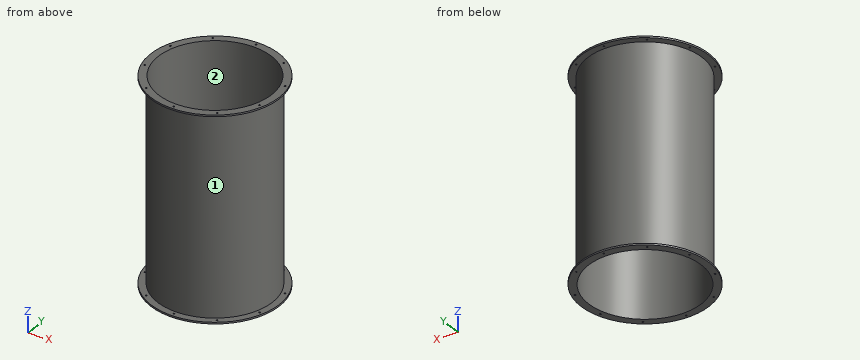
```python
from build123d import *

# Parameters (mm, degrees)
SKETCH1_R           = 425
SKETCH1_R_2         = 419
BOSS_EXTRUDE1_DEPTH = 1500
BOSS_EXTRUDE2_START = -12
SKETCH2_R           = 475
SKETCH2_R_2         = 425
BOSS_EXTRUDE2_DEPTH = 12
SKETCH4_R           = 475
SKETCH4_R_2         = 425
BOSS_EXTRUDE3_DEPTH = 12
SKETCH6_R           = 6
CUT_EXTRUDE3_DEPTH  = 1644.547991389


with BuildPart() as part:
    # Sketch1 → Boss-Extrude1 (new body)
    with BuildSketch(Plane.XY):
        Circle(SKETCH1_R)
        Circle(SKETCH1_R_2, mode=Mode.SUBTRACT)
    extrude(amount=BOSS_EXTRUDE1_DEPTH)

    # Sketch2 → Boss-Extrude2 (add)
    with BuildSketch(Plane.XY.offset(1500).offset(BOSS_EXTRUDE2_START)):
        Circle(SKETCH2_R)
        Circle(SKETCH2_R_2, mode=Mode.SUBTRACT)
    extrude(amount=BOSS_EXTRUDE2_DEPTH)

    # Sketch4 → Boss-Extrude3 (add)
    with BuildSketch(Plane(origin=(0, 0, 0), x_dir=(-1, 0, 0), z_dir=(0, 0, -1))):
        with Locations(Location((0, 0, 0), (0, 0, 180))):
            Circle(SKETCH4_R)
        Circle(SKETCH4_R_2, mode=Mode.SUBTRACT)
    extrude(amount=-BOSS_EXTRUDE3_DEPTH)

    # Sketch6 → Cut-Extrude3 (cut, through all)
    with BuildSketch(Plane.XY.offset(1500)):
        with Locations((0, 450)):
            Circle(SKETCH6_R)
        with Locations((264.503363532, 364.057647469)):
            Circle(SKETCH6_R)
        with Locations((427.975432333, 139.057647469)):
            Circle(SKETCH6_R)
        with Locations((427.975432333, -139.057647469)):
            Circle(SKETCH6_R)
        with Locations((264.503363532, -364.057647469)):
            Circle(SKETCH6_R)
        with Locations((0, -450)):
            Circle(SKETCH6_R)
        with Locations((-264.503363532, -364.057647469)):
            Circle(SKETCH6_R)
        with Locations((-427.975432333, -139.057647469)):
            Circle(SKETCH6_R)
        with Locations((-427.975432333, 139.057647469)):
            Circle(SKETCH6_R)
        with Locations((-264.503363532, 364.057647469)):
            Circle(SKETCH6_R)
    extrude(amount=-CUT_EXTRUDE3_DEPTH, mode=Mode.SUBTRACT)


solid = part.part
```
Could you check a few things on this model? Use its own coordinates, in mm. Face numbers are marked on the shaded views. Round coordinates to 2 decimals unless told otherwise and drop trailing zeros. Loops run counter-clockwise (first coordinate to the right, second up) from the corner with the lowest first, then second, coordinate; pieces in that order, holes last. Notation, with made-up numbers: (23, 61) - (41, 61) arc R23 cw to (41, 71) - close; hole circle Ø1 at (-40, -29). An arc over 180 degrees is marked (long way). Answer in a Markdown table with one row per item. Add a question column.
(1) If we section it at B-B (x = 156): Please give me the cut outline in (y, z).
(2) If we section it at A-A (y = 0): Please give me the cut outline in (x, z).
(3) If we mould it in two halves opening along Y, with no side actions, what happens to the marked faces 1 and 2? For each: pulls with the +Y half, pulls with the -Y half, needs draft (parallel to the pull), parting line crosses it, or undercut.
(4) If we section it at C-C (z = 368): Please give me the cut outline in (x, y).
(5) I'm going to push flat-ended pins straight in: pin 1 (6 mm diameter, centred on y = 157, z = 395, fed in from +X); pin 2 (2 mm diameter, centred on x = -254.5, z = 713.5, fed in from +Y); pin 3 (10 mm diameter, centred on x = -49.5, z = 1231.5, fed in from +Y). Where does each tip first touch, or does it pass through?
(6) I need wall thicknesses on line 1 along Y through (x, z) = (0, 6); line 2 along X through (y, z) = (1, 1132); line 3 along X through (y, z) = (-300, 1389). Which ranges of each line are inside material? Lowest first, please.
Model answer:
| question | item | result |
|---|---|---|
| 1 | outline | (-448.65, 0) - (-388.88, 0) - (-388.88, 1500) - (-448.65, 1500) - (-448.65, 1488) - (-395.33, 1488) - (-395.33, 12) - (-448.65, 12) - close; (388.88, 0) - (448.65, 0) - (448.65, 12) - (395.33, 12) - (395.33, 1488) - (448.65, 1488) - (448.65, 1500) - (388.88, 1500) - close |
| 2 | outline | (-475, 0) - (-419, 0) - (-419, 1500) - (-475, 1500) - (-475, 1488) - (-425, 1488) - (-425, 12) - (-475, 12) - close; (419, 0) - (475, 0) - (475, 12) - (425, 12) - (425, 1488) - (475, 1488) - (475, 1500) - (419, 1500) - close |
| 3 | face 1 | parting line crosses it |
| 3 | face 2 | undercut |
| 4 | outline | circle Ø850 at (0, 0); hole circle Ø838 at (0, 0) |
| 5 | pin 1 | stops at x = 396.12 |
| 5 | pin 2 | stops at y = 341.12 |
| 5 | pin 3 | stops at y = 422.66 |
| 6 | line 1 | y = -475 to -456, -444 to -419, 419 to 444, 456 to 475 |
| 6 | line 2 | x = -425 to -419, 419 to 425 |
| 6 | line 3 | x = -301.04 to -292.51, 292.51 to 301.04 |
